Here's how the part is built. I have some questions about the finished solid (model axes, mm). Face numbers are marked on the shaded views. A direction names the side the tool comes from. Coordinates: 2 decimals unless noted, no trailing zeros. Write each loop counter-clockwise with the first axis right and the second up, starting at its lowest first coordinate (ties: lowest second). Pieces come first, ordered by that corner, then holes. Notation, with made-up numbers: (-6.75, -37.75) -> (17.25, -37.75) arc R22 ccw to (17.25, 0.25) -> close; hole circle Ø5 at (41.25, -5.5). An arc over 180 degrees is marked (long way). Use a Markdown table: item, result. Add a question column.
Item 1: If I drill on line 1 along Z through (x, y) = (4.5, 0); line 2 along Z through (x, y) = (-1.75, 0); line 3 along Z through (x, y) = (-20.5, -1.5), over which ranges is the centre line in solid material (lowest first)? Write a range as from..to.
Item 2: On a 3-axis mill with a long thin cutter (end or side, diameter ignored), from which of +Z, -Z, +X, -X, +Y, -Y can I reach the whole of each face in a straight line? I mean the marked faces 1, 2 and 3. Say none if no direction works.
Item 3: Will these pins go through, and if not, where does the flat tip stop? pin 1 Ø2 at (y, z) = (3.5, -10.5) entering from +X; pin 2 Ø6 at (x, z) = (1.5, -10.5) entering from -Y; pin 3 Ø2 at (y, z) = (-7.5, -1.5) entering from +X; pin 4 Ø2.5 at (x, z) = (-15.5, -1) entering from -Y.
Item 4: Imagine slicing it at C-C, the plane x = -19. Write out the boundary of the cut face in (y, z).
Item 5: Imagine slicing it at A-A, the plane y = 0. Write out the boundary of the cut face in (x, z) (3 decimals), and give its area (3 significant figures).
Item 6: Imagine slicing it at B-B, the plane z = -9.5. Write out the boundary of the cut face in (x, y), and give its area (3 significant figures).
```python
from build123d import *

# Parameters (mm, degrees)
SKETCH1_R                = 10.16
PART_DIA_EXTRUDE_DEPTH   = 16.002
SKETCH1_3_W              = 24.765
SKETCH1_3_H              = 7.8486
ARM_EXTRUDE_DEPTH        = 3.3528
SKETCH2_R                = 6.985
CBORE_EXTRUDE_DEPTH      = 10.2108
SKETCH2_3_R              = 4.1656
THRU_HOLE_EXTRUDE2_DEPTH = 40.737202144
ANGLE_EXTRUDE3_DEPTH     = 40.737202144
FILLET1_R                = 0.254


with BuildPart() as part:
    # Sketch1 → PART DIA EXTRUDE (new body)
    with BuildSketch(Plane.XY):
        Circle(SKETCH1_R)
    extrude(amount=-PART_DIA_EXTRUDE_DEPTH)

    # Sketch1<3> → ARM EXTRUDE (add)
    with BuildSketch(Plane.XY):
        with Locations((-12.3825, 0)):
            Rectangle(SKETCH1_3_W, SKETCH1_3_H)
    extrude(amount=-ARM_EXTRUDE_DEPTH)

    # Sketch2 → CBORE EXTRUDE (cut)
    with BuildSketch(Plane(origin=(10.16, 0, 0), x_dir=(0, 0, -1), z_dir=(1, 0, 0))):
        with Locations((7.983336866, 0)):
            Circle(SKETCH2_R)
    extrude(amount=-CBORE_EXTRUDE_DEPTH, mode=Mode.SUBTRACT)

    # Sketch2<3> → THRU HOLE-Extrude2 (cut, through all)
    with BuildSketch(Plane(origin=(10.16, 0, 0), x_dir=(0, 0, -1), z_dir=(1, 0, 0))):
        with Locations((7.983336866, 0)):
            Circle(SKETCH2_3_R)
    extrude(amount=-THRU_HOLE_EXTRUDE2_DEPTH, mode=Mode.SUBTRACT)

    # Sketch2<4> → ANGLE-Extrude3 (cut, through all)
    with BuildSketch(Plane(origin=(10.16, 0, 0), x_dir=(0, 0, -1), z_dir=(1, 0, 0))):
        Polygon((11.136104206, 10.16), (16.002, 10.16), (16.002, 5.294104206), align=None)
        Polygon((16.002, -10.16), (16.002, -5.294104206), (11.136104206, -10.16), align=None)
    extrude(amount=-ANGLE_EXTRUDE3_DEPTH, mode=Mode.SUBTRACT)

    # Fillet1
    fillet1_edges = [part.edges().sort_by_distance(p)[0] for p in [
        (-10.16, 0, -16.002),
        (0, 5.294104206, -16.002),
        (-5.323615412, 8.653595723, -12.642508482),
        (9.780845679, -2.749665034, -16.002),
        (0, -5.294104206, -16.002),
        (-5.323615412, -8.653595723, -12.642508482),
    ]]
    fillet(fillet1_edges, radius=FILLET1_R)


solid = part.part
```
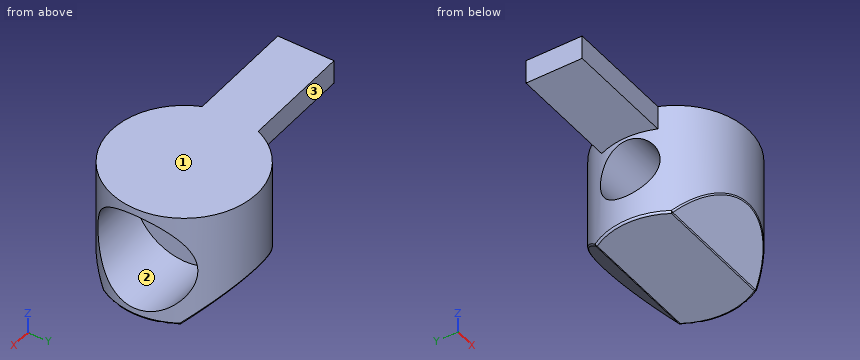
Ans:
| question | item | result |
|---|---|---|
| 1 | line 1 | z = -16..-14.97, -1..0 |
| 1 | line 2 | z = -16..-12.15, -3.82..0 |
| 1 | line 3 | z = -3.35..0 |
| 2 | face 1 | +Z, +X, -X, +Y, -Y |
| 2 | face 2 | +X |
| 2 | face 3 | +Z, -Z, -X, +Y |
| 3 | pin 1 | stops at x = -0.05 |
| 3 | pin 2 | stops at y = -10.16 |
| 3 | pin 3 | stops at x = 7.81 |
| 3 | pin 4 | stops at y = -3.92 |
| 4 | outline | (-3.92, -3.35) -> (3.92, -3.35) -> (3.92, 0) -> (-3.92, 0) -> close |
| 5 | outline | (-24.765, -3.353) -> (-10.16, -3.353) -> (-10.16, -3.818) -> (-0.051, -3.818) -> (-0.051, -0.998) -> (10.16, -0.998) -> (10.16, 0) -> (-24.765, 0) -> close; (-10.16, -15.748) arc R0.254 ccw to (-9.906, -16.002) -> (9.906, -16.002) arc R0.254 ccw to (10.16, -15.748) -> (10.16, -14.968) -> (-0.051, -14.968) -> (-0.051, -12.149) -> (-10.16, -12.149) -> close |
| 5 | area | 147 mm^2 |
| 6 | outline | (-9.39, -3.88) arc R10.16 ccw to (7.53, -6.82) -> (-0.05, -6.82) -> (-0.05, -3.88) -> close; (-9.39, 3.88) -> (-0.05, 3.88) -> (-0.05, 6.82) -> (7.53, 6.82) arc R10.16 ccw to start |
| 6 | area | 120 mm^2 |
